Autodesk Inventor part; units mm, degrees
ref_plane "YZ Plane" through (0, 0, 0) normal (1, 0, 0) x (0, 1, 0)
ref_plane "XZ Plane" through (0, 0, 0) normal (0, 1, 0) x (-1, 0, 0)
ref_plane "XY Plane" through (0, 0, 0) normal (0, 0, 1) x (1, 0, 0)
sketch "Sketch1" plane through (0, 0, 0) normal (0, 1, 0) x (-1, 0, 0)
  line L0 (18.7, 33.5) -> (-17.7, 33.5)
  line L1 (-17.7, 33.5) -> (-17.7, -33.5)
  line L2 (-17.7, -33.5) -> (18.7, -33.5)
  line L3 (18.7, -33.5) -> (18.7, 33.5)
  point P0 (0, 0)
  dimension "d0" = 36.4
  dimension "d1" = 67
extrude "Extrusion1" add sketch "Sketch1" along normal blind 5
sketch "Sketch2" plane through (0, 5, 0) normal (0, 1, 0) x (1, 0, 0)
  line L0 (-18.7, -33.5) -> (17.7, -33.5)
  line L1 (17.7, -33.5) -> (12.7, -33.5)
  line L2 (12.7, -33.5) -> (12.7, -12.5)
  line L3 (12.7, -12.5) -> (17.7, -12.5)
  line L4 (17.7, -12.5) -> (17.7, -33.5)
  line L5 (17.7, -33.5) -> (17.7, 33.5)
  line L6 (17.7, 33.5) -> (12.7, 33.5)
  line L7 (12.7, 33.5) -> (12.7, 12.5)
  line L8 (12.7, 12.5) -> (17.7, 12.5)
  line L9 (17.7, 12.5) -> (17.7, 33.5)
  point P0 (0, 0)
  dimension "d4" = 5
  dimension "d5" = 21
  dimension "d6" = 5
  dimension "d7" = 21
extrude "Extrusion2" add sketch "Sketch2" along normal blind 25.4
sketch "Sketch3" plane through (0, 5, 0) normal (0, 1, 0) x (1, 0, 0)
  circle A0 centre (-0.5, -26) radius 4.25
  circle A1 centre (0, 0) radius 4.25
  circle A2 centre (-0.5, 26) radius 4.25
  line L0 (-18.7, 33.5) -> (-18.7, -33.5)
  dimension "d10" = 8.5
  dimension "d11" = 8.5
  dimension "d12" = 8.5
  dimension "d26" = 18.2
  dimension "d27" = 18.2
extrude "Extrusion3" add sketch "Sketch3" along normal blind 3 contours A0 | A2
sketch "Sketch4" plane through (0, 0, 0) normal (0, -1, 0) x (1, 0, 0)
  circle A0 centre (-0.5, -26) radius 4.25
  circle A1 centre (-0.5, -26) radius 3
  circle A2 centre (-0.5, 26) radius 4.25
  circle A3 centre (-0.5, 26) radius 3
  point P0 (0, 0)
  dimension "d15" = 6
  dimension "d16" = 6
extrude "Extrusion4" cut sketch "Sketch4" against normal blind 3 contours A1 | A3
sketch "Sketch5" plane through (0, 0, 0) normal (0, -1, 0) x (1, 0, 0)
  circle A0 centre (-0.5, -26) radius 3
  circle A1 centre (-0.5, -26) radius 2
  circle A2 centre (-0.5, 26) radius 4.25
  circle A3 centre (-0.5, 26) radius 2
  circle A4 centre (-0.5, 0) radius 2
  point P0 (0, 0)
  dimension "d19" = 4
  dimension "d21" = 4
  dimension "d30" = 4
extrude "Extrusion5" cut sketch "Sketch5" against normal blind 15 contours A1 | A3 | A4
fillet "Fillet1" radius 1.5 2 edges at (-4.75, 8, 26) (-4.75, 8, -26)
fillet "Fillet2" radius 2 6 edges at (-0.5, 0, 33.5) (-18.7, 0, 0) (17.7, 15.2, 33.5) (17.7, 15.2, -33.5) (-0.5, 0, -33.5) (17.7, 0, 0)
properties part number "springBedMount"
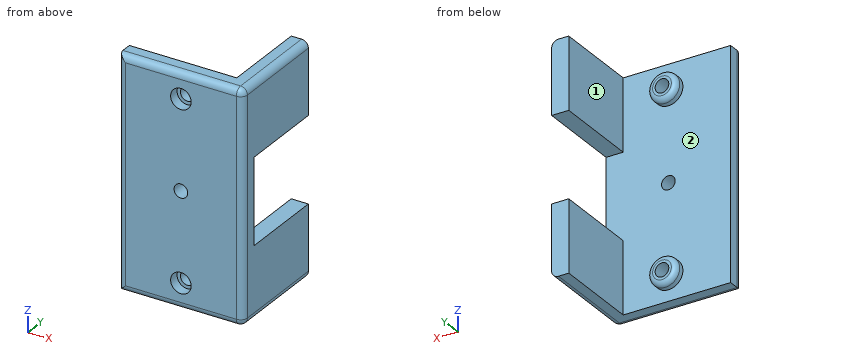
Part model, mm, in its own coordinate system. Face numbers are marked on the shaded views. Round coordinates to 2 decimals unless told otherwise and drop trailing zeros. Loops run counter-clockwise (first coordinate to the right, second up) from the corner with the lowest first, then second, coordinate; pieces in that order, holes last.
Item 1: Cut at A-A, the plane y = 16.5. Give the cut face in (x, z), then the cut area to 3 significant figures.
Item 2: Cut at B-B, the plane z = 0. Give the cut face in (x, y).
Item 3: Cut at C-C, the plane z = -14.5. Give the cut face in (x, y), then the cut area to 3 significant figures.
Item 4: Drop flat-ended pins along their axis: P1, Ø6, axis at x = -1.5, z = -25, coming from the +Y side; P2, Ø5, axis at x = -0.5, z = 26, coming from the -Y side; P3, Ø12, axis at x = -4.5, y = 11.5, coming from the +Z side. Give the stop position or say it passes through.
Item 5: Mould opens along Z. For the marked faces 1 and 2 say: +Z half, -Z half, draft (parallel to the pull), parting line (faces both ways), or undercut.
Item 6: Cut at D-D, the plane x = -10. Give the cut face in (y, z), then the cut area to 3 significant figures.
Item 7: Drill centre lines: line 1 (Z direction, x = -0.5, y = 1.9); line 2 (Z direction, x = 14.5, y = 11); line 3 (Z direction, x = -0.5, y = 0.8). Where is each one in solid material? Low to high.
A:
1. outline: (12.7, -33.5) - (15.7, -33.5) arc R2 ccw to (17.7, -31.5) - (17.7, -12.5) - (12.7, -12.5) - close; (12.7, 12.5) - (17.7, 12.5) - (17.7, 31.5) arc R2 ccw to (15.7, 33.5) - (12.7, 33.5) - close
1. area: 208 mm2
2. outline: (-18.7, 2) arc R2 ccw to (-16.7, 0) - (-2.5, 0) - (-2.5, 5) - (-18.7, 5) - close; (1.5, 0) - (15.7, 0) arc R2 ccw to (17.7, 2) - (17.7, 5) - (1.5, 5) - close
3. outline: (-18.7, 2) arc R2 ccw to (-16.7, 0) - (15.7, 0) arc R2 ccw to (17.7, 2) - (17.7, 30.4) - (12.7, 30.4) - (12.7, 5) - (-18.7, 5) - close
3. area: 307 mm2
4. P1: stops at y = 8
4. P2: stops at y = 3
4. P3: stops at z = 30.22
5. face 1: draft
5. face 2: undercut
6. outline: (0, -31.5) arc R2 ccw to (2, -33.5) - (5, -33.5) - (5, 33.5) - (2, 33.5) arc R2 ccw to (0, 31.5) - close
6. area: 333 mm2
7. line 1: z = -33.5 to -29, -23 to -2, 2 to 23, 29 to 33.5
7. line 2: z = -33.5 to -12.5, 12.5 to 33.5
7. line 3: z = -33.1 to -29, -23 to -2, 2 to 23, 29 to 33.1
